The model under review builds one solid part; all positions refer to its coordinate system, in mm. Face numbers are marked on the shaded views. A direction names the side the tool comes from. Give positions to 0.01 mm unless a question says otherwise; leave off trailing zeros. Order: outer loops, then holes, each group sorted by start corner. A loop starts at its lowest first (then second) coordinate and runs counter-clockwise, first axis right, second up. Notation, with made-up numbers: M 67.5,49.5 L 87.5,49.5 A23 ccw 87.5,76.5 Z; hole C 89.5,-24.75 d4. An arc over 180 degrees is marked long. One line per question, with ' | ' between items. Start each with the question number.
1. We need section A-A on x = 45. Write out the cut boundary in (y, z) (3 decimals).
2. For the marked faces 1, 2, 3 and 4, list the 3-axis set-ups (+Z, -Z, +X, -X, +Y, -Y) from which the entire face can be reached by the end or side of a thin tool; tool diameter is ignored.
3. We need section D-D on x = -25. Write out the cut boundary in (y, z).
4. Insertion check: P1, Ø10, axis at x = 31.5, y = 5.5, coming from the -Z side; P2, Ø10, axis at x = -20.5, z = 5.5, coming from the -Y side; P3, Ø10, axis at y = 10, z = 29.5, coming from the +X side; P4, Ø22, axis at x = 45, z = 45, coming from the +Y side. Each pin has a flat end and moves straight along its axis. Give the tip position at first contact, or say it passes through.
5. We need section B-B on y = 27.5. Write out the cut boundary in (x, z).
6. Wall thickness on L1, parallel to X at y = 1.5, z = -0.5; L2, parallel to X at y = 28, z = -4; L3, parallel to Z at x = 44.5, y = 2.5: over which ranges is each line inside the solid? List them lowest first.
7. We need section C-C on z = 28. Write out the cut boundary in (x, y).
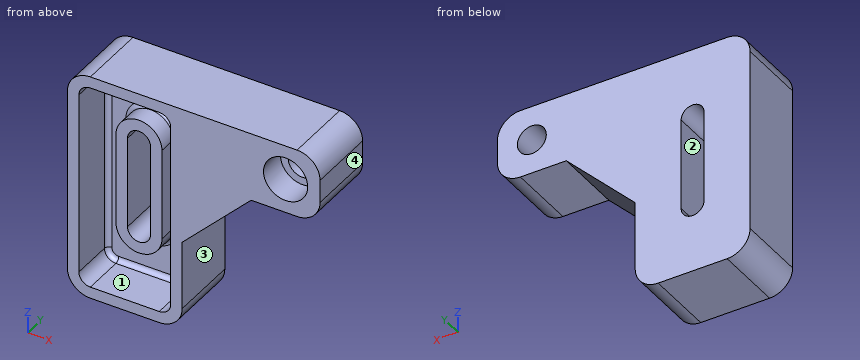
```python
from build123d import *

# Parameters (mm, degrees)
F1_DEPTH       = 30
F2_D           = 12.6
F2_CBORE_D     = 19.25
F2_CBORE_DEPTH = 12
F4_DEPTH       = 20
F7_DEPTH       = 10
F10_DEPTH      = 20.001
F11_R          = 2


with BuildPart() as f1:
    # F0 (on Front) → F1 (new body)
    with BuildSketch(Plane.XZ):
        with BuildLine():
            Line((0, -30), (0, 0))
            Line((0, 0), (30, 30))
            Line((30, 30), (50, 30))
            ThreePointArc((50, 30), (57.0710678119, 32.9289321881), (60, 40))
            Line((60, 40), (60, 50))
            ThreePointArc((60, 50), (57.0710678119, 57.0710678119), (50, 60))
            Line((50, 60), (-40, 60))
            ThreePointArc((-40, 60), (-47.0710678119, 57.0710678119), (-50, 50))
            Line((-50, 50), (-50, -30))
            ThreePointArc((-50, -30), (-47.0710678119, -37.0710678119), (-40, -40))
            Line((-40, -40), (-10, -40))
            ThreePointArc((-10, -40), (-2.9289321881, -37.0710678119), (0, -30))
        make_face()
    extrude(amount=-F1_DEPTH)

    # F2 (through all)
    with Locations(Plane.XZ):
        with Locations((45, 45)):
            CounterBoreHole(F2_D / 2, F2_CBORE_D / 2, F2_CBORE_DEPTH)

    # F3 (on face) → F4 (cut)
    with BuildSketch(Plane.XZ):
        with BuildLine():
            Line((-10, 55), (-40, 55))
            ThreePointArc((-40, 55), (-43.5355339059, 53.5355339059), (-45, 50))
            Line((-45, 50), (-45, -30))
            ThreePointArc((-45, -30), (-43.5355339059, -33.5355339059), (-40, -35))
            Line((-40, -35), (-10, -35))
            ThreePointArc((-10, -35), (-6.4644660941, -33.5355339059), (-5, -30))
            Line((-5, -30), (-5, 50))
            ThreePointArc((-5, 50), (-6.4644660941, 53.5355339059), (-10, 55))
        make_face()
    extrude(amount=-F4_DEPTH, mode=Mode.SUBTRACT)

    # F6 (on offset) → F7 (join)
    with BuildSketch(Plane.XZ.offset(-20)):
        with BuildLine():
            Line((-15, -10), (-15, 30))
            ThreePointArc((-15, 30), (-25, 40), (-35, 30))
            Line((-35, 30), (-35, -10))
            ThreePointArc((-35, -10), (-25, -20), (-15, -10))
        make_face()
    extrude(amount=F7_DEPTH)

    # F9 (on offset) → F10 (cut, through all)
    with BuildSketch(Plane.XZ.offset(-10)):
        with BuildLine():
            Line((-20, -10), (-20, 30))
            ThreePointArc((-20, 30), (-25, 35), (-30, 30))
            Line((-30, 30), (-30, -10))
            ThreePointArc((-30, -10), (-25, -15), (-20, -10))
        make_face()
    extrude(amount=-F10_DEPTH, mode=Mode.SUBTRACT)

    # F11
    f11_edges = [f1.edges().sort_by_distance(p)[0] for p in [
        (-6.464466, 20, 53.535534),
        (-5, 20, 10),
        (-25, 20, 55),
        (-6.464466, 20, -33.535534),
        (-43.535534, 20, 53.535534),
        (-25, 20, -35),
        (-45, 20, 10),
        (-43.535534, 20, -33.535534),
        (-15, 20, 10),
        (-25, 20, 40),
        (-35, 20, 10),
        (-25, 20, -20),
    ]]
    fillet(f11_edges, radius=F11_R)


solid = f1.part
```
Entries:
1) outline: M 0,30 L 30,30 L 30,38.7 L 12,38.7 L 12,35.375 L 0,35.375 Z; M 0,54.625 L 12,54.625 L 12,51.3 L 30,51.3 L 30,60 L 0,60 Z
2) face 1: -Y | face 2: +Y, -Y | face 3: -Z, +X, +Y, -Y | face 4: +Z, -Z, +X, +Y, -Y
3) outline: M 0,-40 L 30,-40 L 30,-15 L 10,-15 L 10,-20 L 18,-20 A2 cw 20,-22 L 20,-33 A2 cw 18,-35 L 0,-35 Z; M 0,55 L 18,55 A2 cw 20,53 L 20,42 A2 cw 18,40 L 10,40 L 10,35 L 30,35 L 30,60 L 0,60 Z
4) P1: stops at z = 26.5 | P2: stops at y = 10 | P3: stops at x = 58.35 | P4: stops at y = 30
5) outline: M -50,-30 A10 ccw -40,-40 L -10,-40 A10 ccw 0,-30 L 0,0 L 30,30 L 50,30 A10 ccw 60,40 L 60,50 A10 ccw 50,60 L -40,60 A10 ccw -50,50 Z; hole M -30,-10 A5 ccw -20,-10 L -20,30 A5 ccw -30,30 Z; hole C 45,45 d12.6
6) L1: x = -50 to -45, -5 to 0 | L2: x = -50 to -30, -20 to 0 | L3: z = 30 to 35.39, 54.61 to 60
7) outline: M -50,0 L -45,0 L -45,18 A2 cw -43,20 L -37,20 A2 cw -35,18 L -35,10 L -30,10 L -30,30 L -50,30 Z; M -20,10 L -15,10 L -15,18 A2 cw -13,20 L -7,20 A2 cw -5,18 L -5,0 L 28,0 L 28,30 L -20,30 Z
